Geometry: final body of the model. Coordinates: model frame, mm. A direction names the side the tool comes from. Coordinates: 2 decimals unless noted, no trailing zeros. Write each loop counter-clockwise with the first axis right and the second up, starting at its lowest first coordinate (ties: lowest second). Pieces come first, ordered by that corner, then holes. Notation, with made-up numbers: M 34,38 L 77,38 A28 cw 77,74 Z; hole C 25.5,47.5 d2. An arc over 180 degrees is marked long. Write item = value, one per line. Start each with the question number.
Item 1: Section B-B on y = 0. Give the number of separate pieces and of enclosed holes in the cut face, plus the area to 3 significant figures.
Item 2: Ray query, L1, parallel to Y at x = 19.5, z = 89; L2, parallel to Y at x = 19.25, z = -72.5; L3, parallel to Y at x = 14, z = 68. Return the intervals inside material, ascending. Write a range as [from, to].
Item 3: Pull-direction query (Z, two-part tool) for faces 3 (the cylindrical face through (24.62, 76.97, -49.07)), 4 (the cylindrical face through (12.522, -9.594, 112.412)), 5 (the flat face through (25.4, 94, -21)), 6 (the cylindrical face through (12.52, 0.14, 117.47)); classes: +Z half, -Z half, draft (parallel to the pull), parting line (faces both ways), or undercut.
Item 4: Section A-A on z = -114.3. Output: boundary loops of the cut face in (x, y) (3 decimals).
Item 5: First-contact query: pin 1 Ø12 at (x, z) = (3.5, -30) entering from -Y; pin 2 Ø4 at (x, z) = (17.5, -47) entering from +Y; pin 3 Ø2 at (x, y) = (15, -11) entering from +Z. Flat tips, straight axial feed; report the tip coordinate or a pass-through.
Item 6: Reachability of faces 1 (the cylindrical face through (24.595, 95.226, 12.503)), 2 (the cylindrical face through (12.52, -102.16, -57.01)) from +Z, -Z, +X, -X, +Y, -Y: full face, straight path, thin tool, end or side. Return the list, or none.
from build123d import *

# Parameters (mm, degrees)
BOSS_EXTRUDE1_START     = -25.4
SKETCH3_R               = 3.175
BOSS_EXTRUDE1_DEPTH     = 25.4
CIRPATTERN1_OUTLINE_R   = 3.175
CIRPATTERN1_OUTLINE_R_2 = 101.6
CIRPATTERN1_DEPTH       = 25.4


with BuildPart() as part:
    # Sketch1 → Revolve1 (revolve)
    with BuildSketch(Plane.XY, mode=Mode.PRIVATE) as revolve1_sk:
        Polygon((0, 111.125), (0, 0), (9.525, 0), (9.525, 82.55), (15.875, 88.9), (25.4, 88.9), (25.4, 98.425), (6.35, 98.425), (6.35, 101.6), (25.4, 101.6), (25.4, 111.125), align=None)
    revolve(revolve1_sk.sketch.rotate(Axis((0, 0, 0), (1, 0, 0)), 90), axis=Axis((0, 0, 0), (1, 0, 0)))

    # Sketch3 → Boss-Extrude1 (add)
    # profile 1 of 3: a face of its own
    with BuildSketch(Plane(origin=(25.4, 0, 0), x_dir=(0, 0, -1), z_dir=(1, 0, 0)).offset(BOSS_EXTRUDE1_START)):
        with BuildLine():
            ThreePointArc((-110.992708333, 5.420730747), (-113.998455884, 6.342836207), (-117.078125, 5.710036907))
            ThreePointArc((-117.078125, 5.710036907), (-120.65, 0), (-117.078125, -5.710036907))
            ThreePointArc((-117.078125, -5.710036907), (-113.998455884, -6.342836207), (-110.992708333, -5.420730747))
            ThreePointArc((-110.992708333, -5.420730747), (-111.09192216, -2.71117239), (-111.125, 0))
            ThreePointArc((-111.125, 0), (-111.09192216, 2.71117239), (-110.992708333, 5.420730747))
        make_face()
        with Locations((-114.3, 0)):
            Circle(SKETCH3_R, mode=Mode.SUBTRACT)
    # profile 2 of 3: a face of its own
    with BuildSketch(Plane(origin=(25.4, 0, 0), x_dir=(0, 0, -1), z_dir=(1, 0, 0)).offset(BOSS_EXTRUDE1_START)):
        with BuildLine():
            ThreePointArc((-110.056490385, 15.373176289), (-112.36034097, 9.664574924), (-117.078125, 5.710036907))
            ThreePointArc((-117.078125, 5.710036907), (-113.998455884, 6.342836207), (-110.992708333, 5.420730747))
            ThreePointArc((-110.992708333, 5.420730747), (-110.636566543, 10.407486174), (-110.056490385, 15.373176289))
        make_face()
    # profile 3 of 3: a face of its own
    with BuildSketch(Plane(origin=(25.4, 0, 0), x_dir=(0, 0, -1), z_dir=(1, 0, 0)).offset(BOSS_EXTRUDE1_START)):
        with BuildLine():
            ThreePointArc((-110.992708333, -5.420730747), (-113.998455884, -6.342836207), (-117.078125, -5.710036907))
            ThreePointArc((-117.078125, -5.710036907), (-112.36034097, -9.664574924), (-110.056490385, -15.373176289))
            ThreePointArc((-110.056490385, -15.373176289), (-110.636566543, -10.407486174), (-110.992708333, -5.420730747))
        make_face()
    extrude(amount=BOSS_EXTRUDE1_DEPTH)

    # CirPattern1: read off the stored shape, not the designer's step
    # CirPattern1 outline → CirPattern1 (add)
    with BuildSketch(Plane.YZ):
        with BuildLine():
            ThreePointArc((-5.710036907, 117.078125), (-9.664574924, 112.36034097), (-15.373176289, 110.056490385))
            ThreePointArc((-15.373176289, 110.056490385), (-55.5625, 96.237072996), (-87.62512838, 68.341806396))
            ThreePointArc((-87.62512838, 68.341806396), (-92.474622196, 64.549937886), (-98.537612024, 63.484099518))
            ThreePointArc((-98.537612024, 63.484099518), (-104.485964967, 60.325), (-104.247648931, 53.594025482))
            ThreePointArc((-104.247648931, 53.594025482), (-102.13919712, 47.810403084), (-102.998304669, 41.714683989))
            ThreePointArc((-102.998304669, 41.714683989), (-111.125, 0), (-102.998304669, -41.714683989))
            ThreePointArc((-102.998304669, -41.714683989), (-102.13919712, -47.810403084), (-104.247648931, -53.594025482))
            ThreePointArc((-104.247648931, -53.594025482), (-104.485964967, -60.325), (-98.537612024, -63.484099518))
            ThreePointArc((-98.537612024, -63.484099518), (-92.474622196, -64.549937886), (-87.62512838, -68.341806396))
            ThreePointArc((-87.62512838, -68.341806396), (-55.5625, -96.237072996), (-15.373176289, -110.056490385))
            ThreePointArc((-15.373176289, -110.056490385), (-9.664574924, -112.36034097), (-5.710036907, -117.078125))
            ThreePointArc((-5.710036907, -117.078125), (0, -120.65), (5.710036907, -117.078125))
            ThreePointArc((5.710036907, -117.078125), (9.664574924, -112.36034097), (15.373176289, -110.056490385))
            ThreePointArc((15.373176289, -110.056490385), (55.5625, -96.237072996), (87.62512838, -68.341806396))
            ThreePointArc((87.62512838, -68.341806396), (92.474622196, -64.549937886), (98.537612024, -63.484099518))
            ThreePointArc((98.537612024, -63.484099518), (104.485964967, -60.325), (104.247648931, -53.594025482))
            ThreePointArc((104.247648931, -53.594025482), (102.13919712, -47.810403084), (102.998304669, -41.714683989))
            ThreePointArc((102.998304669, -41.714683989), (111.125, 0), (102.998304669, 41.714683989))
            ThreePointArc((102.998304669, 41.714683989), (102.13919712, 47.810403084), (104.247648931, 53.594025482))
            ThreePointArc((104.247648931, 53.594025482), (104.485964967, 60.325), (98.537612024, 63.484099518))
            ThreePointArc((98.537612024, 63.484099518), (92.474622196, 64.549937886), (87.62512838, 68.341806396))
            ThreePointArc((87.62512838, 68.341806396), (55.5625, 96.237072996), (15.373176289, 110.056490385))
            ThreePointArc((15.373176289, 110.056490385), (9.664574924, 112.36034097), (5.710036907, 117.078125))
            ThreePointArc((5.710036907, 117.078125), (0, 120.65), (-5.710036907, 117.078125))
        make_face()
        with Locations((-98.986703653, -57.15)):
            Circle(CIRPATTERN1_OUTLINE_R, mode=Mode.SUBTRACT)
        with Locations((0, -114.3)):
            Circle(CIRPATTERN1_OUTLINE_R, mode=Mode.SUBTRACT)
        with Locations((98.986703653, -57.15)):
            Circle(CIRPATTERN1_OUTLINE_R, mode=Mode.SUBTRACT)
        with Locations((-98.986703653, 57.15)):
            Circle(CIRPATTERN1_OUTLINE_R, mode=Mode.SUBTRACT)
        Circle(CIRPATTERN1_OUTLINE_R_2, mode=Mode.SUBTRACT)
        with Locations((98.986703653, 57.15)):
            Circle(CIRPATTERN1_OUTLINE_R, mode=Mode.SUBTRACT)
        with Locations((0, 114.3)):
            Circle(CIRPATTERN1_OUTLINE_R, mode=Mode.SUBTRACT)
    extrude(amount=CIRPATTERN1_DEPTH)

    # Cut-Sweep1: sweep along a path in Sketch4
    with BuildLine(Plane(origin=(25.4, 0, 0), x_dir=(0, 0, -1), z_dir=(1, 0, 0))) as cut_sweep1_path:
        CenterArc((0, 0), 106.3625, 0, 360)
    # Sketch6 → Cut-Sweep1 (sweep, cut)
    with BuildSketch(Plane.XY):
        with BuildLine():
            Line((23.8125, 108.74375), (26.19375, 108.74375))
            Line((26.19375, 108.74375), (26.19375, 103.98125))
            Line((26.19375, 103.98125), (23.8125, 103.98125))
            ThreePointArc((23.8125, 103.98125), (21.43125, 106.3625), (23.8125, 108.74375))
        make_face()
        with BuildLine():
            Line((23.8125, 91.28125), (26.19375, 91.28125))
            Line((26.19375, 91.28125), (26.19375, 96.04375))
            Line((26.19375, 96.04375), (23.8125, 96.04375))
            ThreePointArc((23.8125, 96.04375), (21.43125, 93.6625), (23.8125, 91.28125))
        make_face()
    sweep(path=cut_sweep1_path.line, mode=Mode.SUBTRACT)


solid = part.part
Responses:
q1.separate_pieces = 3
q1.enclosed_holes = 0
q1.area = 2,840 mm²
q2.L1 = [-66.54, -49.01], [-42.03, 42.03], [49.01, 66.54]
q2.L2 = [-84.22, -71.18], [-66.57, -51.45], [51.45, 66.57], [71.18, 84.22]
q2.L3 = [-87.9, -75.49], [-71.16, -54.31], [54.31, 71.16], [75.49, 87.9]
q3.face_3 = undercut
q3.face_4 = +Z half
q3.face_5 = draft
q3.face_6 = undercut
q4.outline = M 0,-7.547 L 25.4,-7.547 L 25.4,-3.175 L 0,-3.175 Z; M 0,3.175 L 25.4,3.175 L 25.4,7.547 L 0,7.547 Z
q5.pin_1 = -108.5
q5.pin_2 = 102.32
q5.pin_3 = 112.12
q6.face_1 = +X
q6.face_2 = +X, -X
